Read the model definition and answer for the solid it produces. Units are mm, in the model's axes. A direction names the side the tool comes from. Give positions to 0.01 mm unless a question says otherwise; leave off trailing zeros. Loops run counter-clockwise (first coordinate to the right, second up) from the corner with the lowest first, then second, coordinate; pieces in that order, holes last. Notation, with made-up numbers: (88.5, 64) - (141.5, 64) arc R34 cw to (141.5, 99) - close; hole circle Ø8 at (-7.75, 51). An arc over 180 degrees is marked (long way). Write item = value, one per line.
```python
from build123d import *

# Parameters (mm, degrees)
BOSS_EXTRUDE1_DEPTH        = 320.675
BOSS_EXTRUDE1_DEPTH_BACK   = 320.675
SKETCH3_W                  = 50.8
SKETCH3_H                  = 25.4
SKETCH3_W_2                = 44.45
SKETCH3_H_2                = 19.05
CUT_EXTRUDE1_DEPTH         = 323.680609311
CUT_EXTRUDE1_DEPTH_BACK    = 323.680609311
F_10_CLEARANCE_HOLE1_D     = 4.9784
F_10_CLEARANCE_HOLE1_DEPTH = 5.08
F_10_CLEARANCE_HOLE1_TIP   = 1.495662253


with BuildPart() as part:
    # Sketch3 → Boss-Extrude1 (new, two sides: drawn at the far end of the back side and taken through both)
    with BuildSketch(Plane.XY.offset(-BOSS_EXTRUDE1_DEPTH_BACK)):
        Rectangle(SKETCH3_W, SKETCH3_H)
        Rectangle(SKETCH3_W_2, SKETCH3_H_2, mode=Mode.SUBTRACT)
    extrude(amount=BOSS_EXTRUDE1_DEPTH + BOSS_EXTRUDE1_DEPTH_BACK)

    # Sketch4 → Cut-Extrude1 (cut, two sides: drawn at the far end of the back side and taken through both)
    with BuildSketch(Plane(origin=(0, 12.7, 0), x_dir=(1, 0, 0), z_dir=(0, 1, 0)).offset(-CUT_EXTRUDE1_DEPTH_BACK)):
        Polygon((1322.117470931, -320.675), (25.4, -320.675), (-25.4, -320.675), (25.4, -305.627354456), (1268.718301677, 62.660305034), (3837.350959621, 420.474595165), (3890.750128875, 37.139290131), align=None)
    extrude(amount=CUT_EXTRUDE1_DEPTH + CUT_EXTRUDE1_DEPTH_BACK, mode=Mode.SUBTRACT)

    # #10 Clearance Hole1
    with Locations(Plane(origin=(0, -12.7, 0), x_dir=(-1, 0, 0), z_dir=(0, -1, 0))):
        with Locations((-11.811, -264.460593775), (11.811, -275.746327933), (-11.811, -297.574221755), (11.811, -308.859955913)):
            Hole(F_10_CLEARANCE_HOLE1_D / 2, depth=F_10_CLEARANCE_HOLE1_DEPTH)
            with Locations((0, 0, -(F_10_CLEARANCE_HOLE1_DEPTH + F_10_CLEARANCE_HOLE1_TIP / 2))):  # 118° drill point
                Cone(0, F_10_CLEARANCE_HOLE1_D / 2, F_10_CLEARANCE_HOLE1_TIP, mode=Mode.SUBTRACT)


solid = part.part
```
1) A cutting plane is placed at A-A on y = 5.25. Determine the outline of the cut face in (x, z) (3 decimals).
Output:
outline = (-25.4, -320.675) - (-22.225, -320.675) - (-22.225, 319.735) - (-25.4, 320.675) - close; (22.225, -320.675) - (25.4, -320.675) - (25.4, 305.627) - (22.225, 306.568) - close
2) A cutting plane is placed at B-B on z = 210. Determine the outline of the cut face in (x, y) (3 decimals), then the cut area to 3 significant figures.
Output:
outline = (-25.4, -12.7) - (25.4, -12.7) - (25.4, 12.7) - (-25.4, 12.7) - close; hole (-22.225, -9.525) - (22.225, -9.525) - (22.225, 9.525) - (-22.225, 9.525) - close
area = 444 mm²
3) A tool of negligible diameter and unlimited length cuts with its end or side. For faces 4 (the face through (25.4, 0, -12)), 5 (the face through (0, -9.525, -5)), from which of +Z, -Z, +X, -X, +Y, -Y can it reach the whole face along a straight path? Write none if from no direction.
Output:
face_4 = +Z, -Z, +X, +Y, -Y
face_5 = +Z, -Z
4) Find the intervals of material crossed by probe 1 along X at (y, z) = (7.25, 65.5) (3 decimals); probe 2 along Y at (x, z) = (5.5, -256) (3 decimals); probe 3 along Z at (x, y) = (6.5, -10) (3 decimals), in increasing order.
Output:
probe_1 = -25.4 to -22.225, 22.225 to 25.4
probe_2 = -12.7 to -9.525, 9.525 to 12.7
probe_3 = -320.675 to 311.226
5) Each of these flat-tipped pins is pushed along its axis until it touches: P1, Ø4, axis at x = 11.81, z = 264.46, coming from the -Y side (3 decimals); P2, Ø6.5, axis at x = 11.81, z = 297.57, coming from the -Y side. Where does it stop, or does it pass through?
Output:
P1 = 9.525
P2 = -12.7
6) The mould has two halves that part along X. Classify faces 1 (the face through (-0.119, -10.407, 313.186)), 2 (the face through (22.225, 0, -11)), 3 (the face through (0, 12.7, -4)): pulls with the +X half, pulls with the -X half, needs draft (parallel to the pull), parting line crosses it, or undercut.
Output:
face_1 = pulls with the +X half
face_2 = undercut
face_3 = needs draft
7) A cutting plane is placed at C-C on x = 4. Determine the outline of the cut face in (y, z) (3 decimals), then the cut area to 3 significant figures.
Output:
outline = (-12.7, -320.675) - (-9.525, -320.675) - (-9.525, 311.966) - (-12.7, 311.966) - close; (9.525, -320.675) - (12.7, -320.675) - (12.7, 311.966) - (9.525, 311.966) - close
area = 4,020 mm²
